```python
from build123d import *

# Parameters (mm, degrees)
BOSS_EXTRUDE1_DEPTH = 208.295833
SKETCH2_W           = 208.295833075
SKETCH2_H           = 125.616174383
CUT_EXTRUDE1_DEPTH  = 20
SKETCH3_R           = 77.5
CUT_EXTRUDE2_DEPTH  = 155.31


with BuildPart() as part:
    # Sketch1 → Boss-Extrude1 (new body)
    with BuildSketch(Plane.XY.offset(413.892285509)):
        Polygon((-272.519046524, -127.125849596), (-268.630033514, -131.644329993), (-324.842905159, -324.071500461), (-330.714338905, -326.339216919), align=None)
    extrude(amount=BOSS_EXTRUDE1_DEPTH)

    # Sketch2 → Cut-Extrude1 (cut)
    with BuildSketch(Plane(origin=(-212.075436587, 61.95263001, 0), x_dir=(0, 0, -1), z_dir=(0.959881544, -0.280405817, 0))):
        with Locations((-518.040202046, -343.17312855)):
            Rectangle(SKETCH2_W, SKETCH2_H)
    extrude(amount=-CUT_EXTRUDE1_DEPTH, mode=Mode.SUBTRACT)

    # Sketch3 → Cut-Extrude2 (cut, through all)
    with BuildSketch(Plane(origin=(0, 0, 568.202285509), x_dir=(-1, 0, 0), z_dir=(0, 0, -1))):
        with Locations((268.126479956, -164.060077585)):
            Circle(SKETCH3_R)
    extrude(amount=CUT_EXTRUDE2_DEPTH, mode=Mode.SUBTRACT)


solid = part.part
```
The model under review builds one solid part; all positions refer to its coordinate system, in mm. Round coordinates to 2 decimals unless told otherwise and drop trailing zeros. Write each loop counter-clockwise with the first axis right and the second up, starting at its lowest first coordinate (ties: lowest second). Pieces come first, ordered by that corner, then holes. Notation, with made-up numbers: (-30, -12.5) -> (11, -12.5) arc R19 cw to (11, 9.5) -> close; hole circle Ø3 at (38.5, -9.5). An arc over 180 degrees is marked (long way). Use CSV: the item, a comma, the result in double quotes.
Q1. Consider section A-A (z = 597.5). Give the boundary of the cut face in (x, y).
Checks:
outline,"(-295.49, -205.76) -> (-290.69, -207.16) -> (-268.63, -131.64) -> (-272.52, -127.13) -> close"
Q2. For pin 1 Ø3 at (y, z) = (-152.5, 616) entering from +X; pin 2 Ø12 at (y, z) = (-186, 611.5) entering from -X; pin 3 Ø10 at (y, z) = (-136, 614) entering from +X; pin 4 Ø6 at (x, y) = (-285.5, -154) entering from -Z, all flat-tipped, find the tip position at first contact; note any pin that passes through.
Checks:
pin 1,"x = -274.28"
pin 2,"x = -291.47"
pin 3,"x = -268.63"
pin 4,"through"
Q3. To check wall thickness, follow probe 1 along X at (y, z) = (-133.5, 604.5); probe 2 along X at (y, z) = (-131, 576.5). State the ranges of each line that lie inside material, in increasing order. Write a range as [from, to].
Checks:
probe 1,"[-274.38, -269.17]"
probe 2,"[-273.65, -269.18]"
Q4. Consider section B-B (x = -285.5). Give the boundary of the cut face in (y, z).
Checks:
outline,"(-189.39, 568.2) -> (-171.56, 568.2) -> (-171.56, 622.19) -> (-189.39, 622.19) -> close"
